Geometry check sheet. Reference: the model listing, model coordinates, mm. A direction names the side the tool comes from. Give positions to 0.01 mm unless a question says otherwise; leave off trailing zeros. Order: outer loops, then holes, each group sorted by start corner. A loop starts at its lowest first (then second) coordinate and runs counter-clockwise, first axis right, second up. Notation, with made-up numbers: M 2.25,-3.75 L 48.25,-3.75 A33 cw 48.25,35.25 Z; hole C 25.5,34 d6. An arc over 180 degrees is marked long. Put each result on its own line as item: value. Start each with the question number.
Q1. Mould release check, pull along Z, two halves, no side actions. Record for faces 6 (the flat face through (-22, -20, 44)), 7 (the flat face through (8.5, 0, -2.7)), 8 (the cylindrical face through (-6.944, -13.804, -5.324)), 9 (the flat face through (0, -22, 15)): +Z half, -Z half, draft (parallel to the pull), parting line (faces both ways), or undercut.
Q2. Go/stop test with flat-tipped pins: pin 1 (8 mm diameter, centred on x = 12.5, z = 29.5, fed in from -Y); pin 2 (6 mm diameter, centred on y = -15.5, z = 4, fed in from +X); pin 3 (1.5 mm diameter, centred on x = 5, y = -22, fed in from +Z). Record where each tip stops, or that it passes through.
Q3. Section check D-D on z = 3.5. Record the cut outline in (x, y).
Q4. Material ranges on L1, parallel to Z at x = 0, y = -21; L2, parallel to Z at x = 0, y = -12; L3, parallel to Y at x = -8, z = 16.5, recorded low to high.
Q5. Section check B-B on z = 29.5. Record the cut outline in (x, y).
Q6. Section check A-A on x = 0. Record the cut outline in (y, z).
Q7. Access from +Z, -Z, +X, -X, +Y, -Y to the whole of each face (thin tool, end or side, straight path). Record for faces 1 (the flat face through (0, -18, 15)), 2 (the cylindrical face through (-10.858, -19.972, 15.214)), 3 (the flat face through (0, -23, 25)), 4 (the cylindrical face through (10.808, -19.972, 14.993)), 5 (the flat face through (0, -17, 25)).
Q8. Section check C-C on y = -4.75. Record the cut outline in (x, z), then the cut area to 3 significant figures.
```python
from build123d import *

# Parameters (mm, degrees)
F0_R     = 8.75
F1_DEPTH = 28
F3_DEPTH = 5
F5_DEPTH = 17
F7_DEPTH = 1
F9_DEPTH = 1


with BuildPart() as f1:
    # F0 (on Front) → F1 (new body)
    with BuildSketch(Plane.XZ):
        with BuildLine():
            ThreePointArc((-12.76405, 2.465566), (-1.238415, -12.940878), (13, 0))
            ThreePointArc((13, 0), (12.940878, 1.238415), (12.76405, 2.465566))
            ThreePointArc((12.76405, 2.465566), (11.670877, 4.703728), (10.906538, 7.07442))
            ThreePointArc((10.906538, 7.07442), (0, 13), (-10.906538, 7.07442))
            ThreePointArc((-10.906538, 7.07442), (-11.670877, 4.703728), (-12.76405, 2.465566))
        make_face()
        Circle(F0_R, mode=Mode.SUBTRACT)
        with BuildLine():
            ThreePointArc((10.906538, 7.07442), (11.670877, 4.703728), (12.76405, 2.465566))
            ThreePointArc((12.76405, 2.465566), (12.057553, 4.85957), (10.906538, 7.07442))
        make_face()
        with BuildLine():
            ThreePointArc((-10.906538, 7.07442), (-12.057553, 4.85957), (-12.76405, 2.465566))
            ThreePointArc((-12.76405, 2.465566), (-11.670877, 4.703728), (-10.906538, 7.07442))
        make_face()
        with BuildLine():
            ThreePointArc((-10.906538, 7.07442), (0, 13), (10.906538, 7.07442))
            ThreePointArc((10.906538, 7.07442), (10.832753, 15.103442), (14.352365, 22.320295))
            ThreePointArc((14.352365, 22.320295), (0, 18), (-14.352365, 22.320295))
            ThreePointArc((-14.352365, 22.320295), (-10.832753, 15.103442), (-10.906538, 7.07442))
        make_face()
        with BuildLine():
            ThreePointArc((-14.352365, 22.320295), (0, 18), (14.352365, 22.320295))
            ThreePointArc((14.352365, 22.320295), (16.553993, 24.567178), (19.122307, 26.383605))
            ThreePointArc((19.122307, 26.383605), (24.21962, 34.544313), (26, 44))
            Line((26, 44), (18, 44))
            ThreePointArc((18, 44), (0, 26), (-18, 44))
            Line((-18, 44), (-26, 44))
            ThreePointArc((-26, 44), (-24.21962, 34.544313), (-19.122307, 26.383605))
            ThreePointArc((-19.122307, 26.383605), (-16.553993, 24.567178), (-14.352365, 22.320295))
        make_face()
        with BuildLine():
            ThreePointArc((19.122307, 26.383605), (16.553993, 24.567178), (14.352365, 22.320295))
            ThreePointArc((14.352365, 22.320295), (16.860191, 24.20773), (19.122307, 26.383605))
        make_face()
        with BuildLine():
            ThreePointArc((-19.122307, 26.383605), (-16.860191, 24.20773), (-14.352365, 22.320295))
            ThreePointArc((-14.352365, 22.320295), (-16.553993, 24.567178), (-19.122307, 26.383605))
        make_face()
    extrude(amount=F1_DEPTH)

    # F2 (on face) → F3 (cut)
    with BuildSketch(Plane.XZ.offset(28)):
        with BuildLine():
            Line((-18, 44), (-26, 44))
            ThreePointArc((-26, 44), (-22.903728, 31.694747), (-14.352365, 22.320295))
            ThreePointArc((-14.352365, 22.320295), (-10.832753, 15.103442), (-10.906538, 7.07442))
            ThreePointArc((-10.906538, 7.07442), (0, 13), (10.906538, 7.07442))
            ThreePointArc((10.906538, 7.07442), (10.832753, 15.103442), (14.352365, 22.320295))
            ThreePointArc((14.352365, 22.320295), (22.903728, 31.694747), (26, 44))
            Line((26, 44), (18, 44))
            ThreePointArc((18, 44), (0, 26), (-18, 44))
        make_face()
    extrude(amount=-F3_DEPTH, mode=Mode.SUBTRACT)

    # F4 (on face) → F5 (cut)
    with BuildSketch(Plane(origin=(0, 0, 0), x_dir=(-1, 0, 0), z_dir=(0, 1, 0))):
        with BuildLine():
            Line((-18, 44), (-26, 44))
            ThreePointArc((-26, 44), (-22.903728, 31.694747), (-14.352365, 22.320295))
            ThreePointArc((-14.352365, 22.320295), (-10.832753, 15.103442), (-10.906538, 7.07442))
            ThreePointArc((-10.906538, 7.07442), (0, 13), (10.906538, 7.07442))
            ThreePointArc((10.906538, 7.07442), (10.832753, 15.103442), (14.352365, 22.320295))
            ThreePointArc((14.352365, 22.320295), (22.903728, 31.694747), (26, 44))
            Line((26, 44), (18, 44))
            ThreePointArc((18, 44), (0, 26), (-18, 44))
        make_face()
    extrude(amount=-F5_DEPTH, mode=Mode.SUBTRACT)

    # F6 (on face) → F7 (cut)
    with BuildSketch(Plane(origin=(0, -17, 0), x_dir=(-1, 0, 0), z_dir=(0, 1, 0))):
        with BuildLine():
            ThreePointArc((14.352365, 22.320295), (0, 18), (-14.352365, 22.320295))
            ThreePointArc((-14.352365, 22.320295), (-10.832753, 15.103442), (-10.906538, 7.07442))
            ThreePointArc((-10.906538, 7.07442), (0, 13), (10.906538, 7.07442))
            ThreePointArc((10.906538, 7.07442), (10.832753, 15.103442), (14.352365, 22.320295))
        make_face()
    extrude(amount=-F7_DEPTH, mode=Mode.SUBTRACT)

    # F8 (on face) → F9 (cut)
    with BuildSketch(Plane.XZ.offset(23)):
        with BuildLine():
            ThreePointArc((14.352365, 22.320295), (0, 18), (-14.352365, 22.320295))
            ThreePointArc((-14.352365, 22.320295), (-10.832753, 15.103442), (-10.906538, 7.07442))
            ThreePointArc((-10.906538, 7.07442), (0, 13), (10.906538, 7.07442))
            ThreePointArc((10.906538, 7.07442), (10.832753, 15.103442), (14.352365, 22.320295))
        make_face()
    extrude(amount=-F9_DEPTH, mode=Mode.SUBTRACT)


solid = f1.part
```
Results found:
1. face 6: +Z half
1. face 7: draft
1. face 8: undercut
1. face 9: undercut
2. pin 1: stops at y = -23
2. pin 2: stops at x = 12.96
2. pin 3: stops at z = 26.94
3. outline: M -12.52,-28 L -8.02,-28 L -8.02,0 L -12.52,0 Z; M 8.02,-28 L 12.52,-28 L 12.52,0 L 8.02,0 Z
4. L1: z = -13 to -8.75, 8.75 to 26
4. L2: z = -13 to -8.75, 8.75 to 13
4. L3: y = -22 to -18
5. outline: M -21.58,-23 L -10.67,-23 L -10.67,-17 L -21.58,-17 Z; M 10.67,-23 L 21.58,-23 L 21.58,-17 L 10.67,-17 Z
6. outline: M -28,-13 L 0,-13 L 0,-8.75 L -28,-8.75 Z; M -28,8.75 L 0,8.75 L 0,13 L -18,13 L -18,18 L -17,18 L -17,26 L -23,26 L -23,18 L -22,18 L -22,13 L -28,13 Z
7. face 1: +Y
7. face 2: -X, +Y, -Y
7. face 3: +Z, +X, -X, -Y
7. face 4: +X, +Y, -Y
7. face 5: +Z, +X, -X, +Y
8. outline: M -12.76,2.47 A13 ccw long 13,0 A13 ccw 12.76,2.47 A13 ccw 10.91,7.07 A13 ccw -10.91,7.07 A13 ccw Z; hole C 0,0 d17.5
8. area: 290 mm^2
